Could you check a few things on this model? Use its own coordinates, in mm. A direction names the side the tool comes from. Round coordinates to 2 decimals unless told otherwise and drop trailing zeros. Loops run counter-clockwise (first coordinate to the right, second up) from the corner with the lowest first, then second, coordinate; pieces in that order, holes last. Notation, with made-up numbers: M 45,70 L 56,70 A16 cw 56,93 Z; hole C 77.25,0.25 d4. An arc over 180 degrees is marked long. Return JSON: item names as keys, results as strings. Group by question number.
```python
from build123d import *

# Parameters (mm, degrees)
SKETCH2_W            = 47.895999966
SKETCH2_H            = 27.94
BOSS_EXTRUDE1_DEPTH  = 2.54
SKETCH4_W            = 6.604
SKETCH4_H            = 2.54
BOSS_EXTRUDE7_DEPTH  = 22.86
SKETCH22_W           = 41.291999966
SKETCH22_H           = 2.54
BOSS_EXTRUDE9_DEPTH  = 10.16
SKETCH23_W           = 7.62
SKETCH23_H           = 2.54
BOSS_EXTRUDE10_DEPTH = 6.604
SKETCH24_W           = 7.62
SKETCH24_H           = 2.54
BOSS_EXTRUDE11_DEPTH = 6.604
CUT_EXTRUDE2_DEPTH   = 6.604
SKETCH26_R           = 1.75
CUT_EXTRUDE3_DEPTH   = 6.604
SKETCH28_W           = 0.381
SKETCH28_H           = 20.32
CUT_EXTRUDE4_DEPTH   = 6.604
SKETCH29_W           = 47.895999966
SKETCH29_H           = 2.54
BOSS_EXTRUDE12_DEPTH = 5.08
SKETCH31_W           = 3.81
SKETCH31_H           = 10.853375152
BOSS_EXTRUDE13_DEPTH = 22.86
SKETCH32_W           = 3.81
SKETCH32_H           = 33.02
BOSS_EXTRUDE14_DEPTH = 33.02
SKETCH33_R           = 5
SKETCH33_R_2         = 1
CUT_EXTRUDE5_DEPTH   = 9.144
SKETCH34_R           = 11
CUT_EXTRUDE6_DEPTH   = 9.144
FILLET6_R            = 2.54
FILLET7_R            = 3.81
BOSS_EXTRUDE15_DEPTH = 2.54


with BuildPart() as part:
    # Sketch2 → Boss-Extrude1 (new body)
    with BuildSketch(Plane(origin=(0, 0, 0), x_dir=(1, 0, 0), z_dir=(0, 1, 0))):
        with Locations((-1397.315525756, 385.150412371)):
            Rectangle(SKETCH2_W, SKETCH2_H)
    extrude(amount=BOSS_EXTRUDE1_DEPTH)

    # Sketch4 → Boss-Extrude7 (add)
    with BuildSketch(Plane.XZ):
        with Locations((-1424.565525739, -400.390412371)):
            Rectangle(SKETCH4_W, SKETCH4_H)
        with Locations((-1376.669525773, -400.390412371)):
            Rectangle(SKETCH4_W, SKETCH4_H)
    extrude(amount=-BOSS_EXTRUDE7_DEPTH)


with BuildPart() as boss_extrude7_piece_1:
    # of the separate pieces the step leaves, piece 1, a body of its own (boss_extrude7_pieces)
    add(part.part.solids().sort_by_distance((-1379.971525773, 0, -399.120412371))[0])



with BuildPart() as boss_extrude7_piece_2:
    # of the separate pieces the step leaves, piece 2, a body of its own (boss_extrude7_pieces)
    add(part.part.solids().sort_by_distance((-1421.263525739, 22.86, -399.120412371))[0])


with BuildPart() as boss_extrude7_piece_1_1:
    add(boss_extrude7_piece_1.part)

    add(boss_extrude7_piece_2.part)  # Boss-Extrude9 merges Boss-Extrude7 piece 2
    # Sketch22 → Boss-Extrude9 (add)
    with BuildSketch(Plane(origin=(0, 0, -399.120412371), x_dir=(-1, 0, 0), z_dir=(0, 0, -1))):
        with Locations((1400.617525756, 1.27)):
            Rectangle(SKETCH22_W, SKETCH22_H)
    extrude(amount=BOSS_EXTRUDE9_DEPTH)

    # Sketch23 → Boss-Extrude10 (add)
    with BuildSketch(Plane(origin=(-1379.971525773, 0, 0), x_dir=(0, 0, -1), z_dir=(1, 0, 0))):
        with Locations((405.470412371, 1.27)):
            Rectangle(SKETCH23_W, SKETCH23_H)
    extrude(amount=BOSS_EXTRUDE10_DEPTH)

    # Sketch24 → Boss-Extrude11 (add)
    with BuildSketch(Plane.ZY.offset(1421.263525739)):
        with Locations((-405.470412371, 1.27)):
            Rectangle(SKETCH24_W, SKETCH24_H)
    extrude(amount=BOSS_EXTRUDE11_DEPTH)

    # Sketch25 → Cut-Extrude2 (cut)
    with BuildSketch(Plane(origin=(0, 2.54, 0), x_dir=(1, 0, 0), z_dir=(0, 1, 0))):
        with BuildLine():
            Line((-1420.553753649, 409.280412371), (-1427.867525739, 409.280412371))
            Line((-1427.867525739, 409.280412371), (-1427.867525739, 401.660412371))
            ThreePointArc((-1427.867525739, 401.660412371), (-1423.137532321, 404.440430382), (-1420.553753649, 409.280412371))
        make_face()
        with BuildLine():
            Line((-1379.971525773, 409.280412371), (-1373.367525773, 409.280412371))
            Line((-1373.367525773, 409.280412371), (-1373.367525773, 401.660412371))
            ThreePointArc((-1373.367525773, 401.660412371), (-1378.247679446, 404.102679188), (-1379.971525773, 409.280412371))
        make_face()
    extrude(amount=-CUT_EXTRUDE2_DEPTH, mode=Mode.SUBTRACT)

    # Sketch26 → Cut-Extrude3 (cut)
    with BuildSketch(Plane.XY.offset(-399.120412371)):
        with Locations((-1424.617525739, 17.61)):
            Circle(SKETCH26_R)
        with Locations((-1424.617525739, 7.61)):
            Circle(SKETCH26_R)
        with Locations((-1376.721525773, 18.514296447)):
            Circle(SKETCH26_R)
        with Locations((-1376.721525773, 8.514296447)):
            Circle(SKETCH26_R)
    extrude(amount=-CUT_EXTRUDE3_DEPTH, mode=Mode.SUBTRACT)

    # Sketch28 → Cut-Extrude4 (cut)
    with BuildSketch(Plane.XY.offset(-399.120412371)):
        with Locations((-1421.454025739, 12.7)):
            Rectangle(SKETCH28_W, SKETCH28_H)
    extrude(amount=-CUT_EXTRUDE4_DEPTH, mode=Mode.SUBTRACT)

    # Sketch29 → Boss-Extrude12 (add)
    with BuildSketch(Plane.XY.offset(-371.180412371)):
        with Locations((-1397.315525756, 1.27)):
            Rectangle(SKETCH29_W, SKETCH29_H)
    extrude(amount=BOSS_EXTRUDE12_DEPTH)

    # Sketch31 → Boss-Extrude13 (add)
    with BuildSketch(Plane.XZ):
        Polygon((-1421.263525739, -366.100412371), (-1373.367525773, -366.100412371), (-1373.367525773, -362.290412371), (-1433.057525773, -362.290412371), (-1436.867525773, -362.290412371), (-1436.867525773, -366.100412371), align=None)
        with Locations((-1434.962525773, -356.863724795)):
            Rectangle(SKETCH31_W, SKETCH31_H)
        Polygon((-1436.867525773, -351.437037219), (-1433.057525773, -351.437037219), (-1433.057525773, -347.627037219), (-1445.757525773, -347.627037219), (-1445.757525773, -351.437037219), align=None)
    extrude(amount=-BOSS_EXTRUDE13_DEPTH)

    # Sketch32 → Boss-Extrude14 (add)
    with BuildSketch(Plane.ZY.offset(1445.757525773)):
        with Locations((-349.532037219, 11.43)):
            Rectangle(SKETCH32_W, SKETCH32_H)
    extrude(amount=BOSS_EXTRUDE14_DEPTH)

    # Sketch33 → Cut-Extrude5 (cut)
    with BuildSketch(Plane.XY.offset(-362.290412371)):
        with Locations((-1402.577525773, 11.43)):
            Circle(SKETCH33_R)
        with Locations((-1412.577525773, 11.43)):
            Circle(SKETCH33_R_2)
        with Locations((-1392.577525773, 11.43)):
            Circle(SKETCH33_R_2)
    extrude(amount=-CUT_EXTRUDE5_DEPTH, mode=Mode.SUBTRACT)

    # Sketch34 → Cut-Extrude6 (cut)
    with BuildSketch(Plane.XY.offset(-347.627037219)):
        with Locations((-1462.267525773, 11.43)):
            Circle(SKETCH34_R)
    extrude(amount=-CUT_EXTRUDE6_DEPTH, mode=Mode.SUBTRACT)

    # Fillet6
    fillet6_edges = [boss_extrude7_piece_1_1.edges().sort_by_distance(p)[0] for p in [
        (-1421.263525739, 1.27, -366.100412371),
        (-1436.867525773, 11.43, -366.100412371),
        (-1436.867525773, 11.43, -351.437037219),
        (-1433.057525773, 11.43, -347.627037219),
        (-1433.057525773, 11.43, -362.290412371),
        (-1373.367525773, 22.86, -364.195412371),
    ]]
    fillet(fillet6_edges, radius=FILLET6_R)

    # Fillet7
    fillet7_edges = [boss_extrude7_piece_1_1.edges().sort_by_distance(p)[0] for p in [
        (-1445.757525773, -5.08, -349.532037219),
        (-1445.757525773, 27.94, -349.532037219),
        (-1478.777525773, -5.08, -349.532037219),
        (-1478.777525773, 27.94, -349.532037219),
    ]]
    fillet(fillet7_edges, radius=FILLET7_R)

    # Sketch35 → Boss-Extrude15 (add)
    with BuildSketch(Plane(origin=(0, 2.54, 0), x_dir=(1, 0, 0), z_dir=(0, 1, 0))):
        with BuildLine():
            Line((-1421.263525739, 399.120412371), (-1421.771525739, 399.120412371))
            ThreePointArc((-1421.771525739, 399.120412371), (-1421.412315494, 398.971622616), (-1421.263525739, 398.612412371))
            Line((-1421.263525739, 398.612412371), (-1421.263525739, 399.120412371))
        make_face()
    extrude(amount=-BOSS_EXTRUDE15_DEPTH)


solid = boss_extrude7_piece_1_1.part
```
1. If we section it at D-D, the plane x = -1447: Please give me the cut outline in (y, z), then the cut area to 3 significant figures.
2. I'm going to push flat-ended pins straight in: pin 1 Ø5.5 at (x, y) = (-1424.62, 17.61) entering from -Z; pin 2 Ø6 at (x, y) = (-1448.5, 24) entering from -Z; pin 3 Ø13 at (x, z) = (-1390.5, -392.5) entering from +Y; pin 4 Ø9 at (x, z) = (-1414.5, -354) entering from +Y. Where does each tip first touch, or does it pass through?
3. I need wall thicknesses on probe 1 along X at (y, z) = (3, -401); probe 2 along Z at (x, y) = (-1412, 22); probe 3 along X at (y, z) = (11.5, -359). Which ranges of each line are inside material? Lowest first, please.
4. If we section it at A-A, the plane y = 14.5: Please give me the cut outline in (x, z).
5. If we section it at B-B, the plane z = -372.5: Please give me the cut outline in (x, y).
6. On a 3-axis mill with a long thin cutter (end or side, diameter ignored), from which of +Z, -Z, +X, -X, +Y, -Y can I reach the whole of each face in a straight line? I mean faces 5 (the face through (-1425, 13, -401.66)), 6 (the face through (-1379.972, 13, -400)), 7 (the face through (-1422.03, 1.29, -366.82)), 8 (the face through (-1375.052, 9.04, -400.373)). Say none if no direction works.
7. If we section it at C-C, the plane x = -1417: Please give me the cut outline in (y, z).
8. We'd pull the mould along Y, two halves only. Please class faces 1 (the face through (-1436.14, 11.59, -365.34)), 2 (the face through (-1477.632, 26.854, -349.505)), 3 (the face through (-1411.624, 11.73, -364.169)), 4 (the face through (-1375.052, 19.04, -400.373)): +Y half, -Y half, draft (parallel to the pull), parting line (faces both ways), or undercut.
Geometry results:
{
 "1": {"outline": "M -4.08,-351.44 L 26.94,-351.44 L 26.94,-347.63 L -4.08,-347.63 Z", "area": "118 mm^2"},
 "2": {"pin 1": "z = -401.66", "pin 2": "z = -351.44", "pin 3": "y = 2.54", "pin 4": "through"},
 "3": {"probe 1": "-1427.87 to -1421.64, -1379.97 to -1373.37", "probe 2": "-366.1 to -362.29", "probe 3": "-1436.87 to -1433.06"},
 "4": {"outline": "M -1478.78,-351.44 L -1472.83,-351.44 L -1472.83,-347.63 L -1478.78,-347.63 Z; M -1451.7,-351.44 L -1439.41,-351.44 A2.54 cw -1436.87,-353.98 L -1436.87,-363.56 A2.54 ccw -1434.33,-366.1 L -1406.52,-366.1 L -1406.52,-362.29 L -1430.52,-362.29 A2.54 cw -1433.06,-359.75 L -1433.06,-350.17 A2.54 ccw -1435.6,-347.63 L -1451.7,-347.63 Z; M -1427.87,-401.66 L -1421.64,-401.66 L -1421.64,-399.12 L -1427.87,-399.12 Z; M -1398.63,-366.1 L -1373.37,-366.1 L -1373.37,-362.29 L -1398.63,-362.29 Z; M -1379.97,-401.66 L -1373.37,-401.66 L -1373.37,-399.12 L -1379.97,-399.12 Z"},
 "5": {"outline": "M -1421.26,0 L -1373.37,0 L -1373.37,2.54 L -1421.26,2.54 Z"},
 "6": {"face 5": "-Z, +X, -X, +Y", "face 6": "-Z, +Y", "face 7": "-X, +Y, -Y", "face 8": "-Z"},
 "7": {"outline": "M 0,-409.28 L 2.54,-409.28 L 2.54,-366.1 L 22.86,-366.1 L 22.86,-362.29 L 0,-362.29 Z"},
 "8": {"face 1": "draft", "face 2": "+Y half", "face 3": "undercut", "face 4": "undercut"}
}
